Source: CAD feature listing. Evaluate the final solid. Frame: model axes, mm. Give positions to 0.01 mm unless a question says otherwise; leave off trailing zeros. Loops run counter-clockwise (first coordinate to the right, second up) from the corner with the lowest first, then second, coordinate; pieces in that order, holes last. Notation, with made-up numbers: (43, 15.5) -> (76, 15.5) arc R16 cw to (76, 19.5) -> close; hole circle Ø5 at (-22.5, -23.5). An arc over 180 degrees is marked (long way). Return JSON: item names as keys, results as strings. Group by question number.
(1) Ray query, line 1 (X direction, y = -0.25, z = 6.75); line 2 (Y direction, x = 37.05, z = 9.25); line 3 (Z direction, x = 37, y = -2) (3 decimals). Return the intervals inside material, ascending. Write a range as from..to.
(2) Cut plane B-B on z = 5.25. Return loops of the section in (x, y).
(3) Cut plane C-C on x = 36.4. Return loops of the section in (y, z) (3 decimals).
(4) Draft query along Z for faces 1 (the face through (35.72, 0.12, 6.17)), 2 (the face through (35.454, 0.094, 6.31)). Return one class per face: released by +Z, released by -Z, zero draft, split by the parting line, or undercut.
```python
from build123d import *

# Parameters (mm, degrees)
PAD003_DEPTH    = 0.3
SKETCH013_W     = 6.14
SKETCH013_H     = 0.25
POCKET009_DEPTH = 0.001
POCKET010_DEPTH = 0.001


with BuildPart() as part:
    # Sketch012 (on Face1 of Binder003) → Pad003 (new body)
    with BuildSketch(Plane(origin=(25.7763153586, 0, -13.2186232608), x_dir=(0, -1, 0), z_dir=(-0.8898174628, 0, 0.4563166476))):
        with BuildLine():
            Line((-3.1497057125, 24.5214914082), (-3.1497057125, 18.9611513515))
            ThreePointArc((-3.1497057125, 18.9611513515), (-2.9388225949, 18.452034469), (-2.4297057125, 18.2411513515))
            Line((-2.4297057125, 18.2411513515), (2.2702942875, 18.2411513515))
            ThreePointArc((2.2702942875, 18.2411513515), (2.77941117, 18.452034469), (2.9902942875, 18.9611513515))
            Line((2.9902942875, 18.9611513515), (2.9902942875, 24.5214914082))
            ThreePointArc((2.9902942875, 24.5214914082), (2.77941117, 25.0306082907), (2.2702942875, 25.2414914082))
            Line((2.2702942875, 25.2414914082), (-2.4297057125, 25.2414914082))
            ThreePointArc((-2.4297057125, 25.2414914082), (-2.9388225949, 25.0306082907), (-3.1497057125, 24.5214914082))
        make_face()
    extrude(amount=PAD003_DEPTH)

    # Sketch013 (on Face10 of Pad003) → Pocket009 (cut)
    with BuildSketch(Plane(origin=(25.5093701197, 0, -13.0817282665), x_dir=(0, -1, 0), z_dir=(-0.8898174628, 0, 0.4563166476))):
        with Locations((-0.0797057125, 19.748978)):
            Rectangle(SKETCH013_W, SKETCH013_H)
        with Locations((-0.0797057125, 18.698219)):
            Rectangle(SKETCH013_W, SKETCH013_H)
        with Locations((-0.0797057125, 20.86224)):
            Rectangle(SKETCH013_W, SKETCH013_H)
    extrude(amount=-POCKET009_DEPTH, mode=Mode.SUBTRACT)

    # Sketch014 (on Face12 of Pocket009) → Pocket010 (cut)
    with BuildSketch(Plane(origin=(25.5093701197, 0, -13.0817282665), x_dir=(0, -1, 0), z_dir=(-0.8898174628, 0, 0.4563166476))):
        Polygon((-1.0997057125, 20.98724), (-1.3497057125, 20.98724), (-0.0797057125, 23.55931), (1.1902942875, 20.98724), (0.9402942875, 20.98724), (-0.0797057125, 23.022278), align=None)
    extrude(amount=-POCKET010_DEPTH, mode=Mode.SUBTRACT)


solid = part.part
```
Answers:
{
 "1": {"line 1": "35.68..36.02", "line 2": "-2.64..2.8", "line 3": "8.668..9.325"},
 "2": {"outline": "(34.91, -2.99) -> (35.25, -2.99) -> (35.25, 3.15) -> (34.91, 3.15) -> close"},
 "3": {"outline": "(-2.99, 7.498) -> (3.15, 7.498) -> (3.15, 8.155) -> (-2.99, 8.155) -> close"},
 "4": {"face 1": "released by -Z", "face 2": "released by +Z"}
}
